from build123d import *

# Parameters (mm, degrees)
BOSS_EXTRUDE1_DEPTH = 57.15
BOSS_EXTRUDE2_REACH = 65.5
CUT_EXTRUDE1_REACH  = 52.8
SKETCH4_W           = 76.2
SKETCH4_H           = 7.9375


with BuildPart() as part:
    # Sketch2 → Boss-Extrude1 (new body, symmetric)
    with BuildSketch(Plane(origin=(0, 0, 0), x_dir=(0, 0, -1), z_dir=(1, 0, 0))):
        Polygon((-63.5, 0), (0, 0), (0, 50.8), (-15.875, 50.8), (-47.625, 12.7), (-63.5, 12.7), align=None)
    extrude(amount=BOSS_EXTRUDE1_DEPTH, both=True)

    # Sketch3 → Boss-Extrude2 (add, up to next)
    with BuildSketch(Plane.XY.offset(63.5), mode=Mode.PRIVATE) as boss_extrude2_sk1:
        Polygon((-44.45, 12.7), (44.45, 12.7), (0, 38.363219465), align=None)
    boss_extrude2_tool1 = extrude(boss_extrude2_sk1.sketch, amount=-BOSS_EXTRUDE2_REACH, mode=Mode.PRIVATE) - part.part
    add(boss_extrude2_tool1.solids().sort_by_distance((0, 21.254406, 63.5))[0])

    # Sketch4 → Cut-Extrude1 (cut, up to next)
    with BuildSketch(Plane(origin=(0, 50.8, 0), x_dir=(1, 0, 0), z_dir=(0, 1, 0)), mode=Mode.PRIVATE) as cut_extrude1_sk1:
        with Locations((0, -3.96875)):
            Rectangle(SKETCH4_W, SKETCH4_H)
    cut_extrude1_tool1 = extrude(cut_extrude1_sk1.sketch, amount=-CUT_EXTRUDE1_REACH, mode=Mode.PRIVATE) & part.part
    add(cut_extrude1_tool1.solids().sort_by_distance((0, 50.8, 3.96875))[0], mode=Mode.SUBTRACT)


solid = part.part
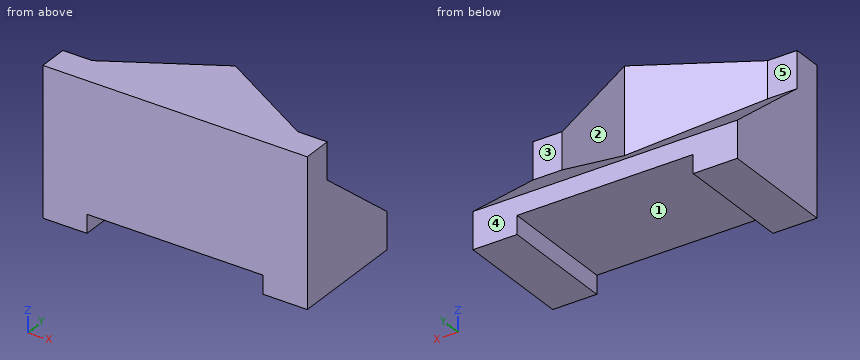
Could you check a few things on this model? Use its own coordinates, in mm. Face numbers are marked on the shaded views. A direction names the side the tool comes from. Coordinates: 2 decimals unless noted, no trailing zeros. Loops run counter-clockwise (first coordinate to the right, second up) from the corner with the lowest first, then second, coordinate; pieces in that order, holes last.
1. Imagine slicing it at B-B (z = 29). Please give me the cut outline in (x, y), and give its area (3 significant figures).
2. For the marked faces 4 and 5, which set-ups out of +Z, -Z, +X, -X, +Y, -Y let a thin tool reach every point of the face, with its end or its side?
3. I need wall thicknesses on L1, parallel to X at y = 39, z = 7.5; L2, parallel to Z at x = 19, y = 20; L3, parallel to Y at x = 3, z = 47. Which ranges of each line are inside material? Lowest first, please.
4. Imagine slicing it at D-D (z = 17.5). Please give me the cut outline in (x, y), and give its area (3 significant figures).
5. Imagine slicing it at C-C (x = -4). Please give me the cut outline in (y, z) (1 decimal).
6. We'd pull the mould along X, two halves only. Please class the marked faces 1, 2 and 3: released by +X, released by -X, zero draft, split by the parting line, or undercut.
7. For P1, Ø10, axis at x = 33, y = 42, coming from the -Z side; P2, Ø4, axis at y = 31.5, z = 57, coming from the -X side; P3, Ø14, axis at x = 48.5, z = 55.5, coming from the +Y side, each with a flat end and sliding along its axis, tell me the tip position at first contact or that it passes through.
Computed values:
1. outline: (-57.15, 0) - (57.15, 0) - (57.15, 35.05) - (5.74, 35.05) - (0, 38.36) - (-5.74, 35.05) - (-57.15, 35.05) - close
1. area: 4,030 mm2
2. face 4: +Z, -Z, +X, -X, +Y
2. face 5: +Z, -X, +Y
3. L1: x = -57.15 to -38.1, 38.1 to 57.15
3. L2: z = 7.94 to 63.5
3. L3: y = 0 to 36.63
4. outline: (-57.15, 0) - (57.15, 0) - (57.15, 48.85) - (-57.15, 48.85) - close
4. area: 5,580 mm2
5. outline: (0, 7.9) - (50.8, 7.9) - (50.8, 15.9) - (36.1, 28.2) - (36.1, 63.5) - (0, 63.5) - close
6. face 1: undercut
6. face 2: released by +X
6. face 3: zero draft
7. P1: stops at z = 7.94
7. P2: stops at x = -15.35
7. P3: stops at y = 14.4
